The listing builds one solid part. Answer for the finished solid, in the listing's coordinates (mm). A direction names the side the tool comes from. Round coordinates to 2 decimals unless told otherwise and drop trailing zeros. Order: outer loops, then holes, each group sorted by start corner. A loop starts at its lowest first (then second) coordinate and runs counter-clockwise, first axis right, second up. Notation, with made-up numbers: (26.5, 48.25) - (68.5, 48.25) arc R15 ccw to (68.5, 75.25) - close; hole circle Ø9 at (49, 51). An arc over 180 degrees is marked (long way). Use CSV: the item, a comma, the result in double quotes. Start each with the question number.
Item 1: For faces 4 (the flat face through (-1, 53, 2)), 5 (the flat face through (58.1, 4.5, 4.7)), 6 (the flat face through (118, 2, 2)), determine the directions among +Z, -Z, +X, -X, +Y, -Y from which every point of the face is accessible in a straight line to the end or side of a thin tool.
Item 2: Flat-ended cylindrical pins translate along their axes: P1, Ø1, axis at y = 54, z = 1.5, coming from the -X side; P2, Ø2, axis at x = 74, z = 3.5, coming from the +Y side; P3, Ø5, axis at y = 9.5, z = 6, coming from the -X side; P4, Ø8, axis at x = 76, y = 16.5, coming from the -Z side. Find the tip coordinate at first contact, or state that the pin passes through.
Item 3: Determine the mould class of faces 1 (the cylindrical face through (0.738, 53.523, 0.986)), 2 (the flat face through (64, 9, 2)), 3 (the flat face through (53, 8, 24)) for opening direction Z: +Z half, -Z half, draft (parallel to the pull), parting line (faces both ways), or undercut.
Item 4: Find section B-B, the plane x = 93. Give the vertices of the cut face in (y, z), plus the area to 3 significant figures.
Item 5: Find section A-A, the plane y = 31.5. Give the vertices of the cut face in (x, z).
Item 6: Find section C-C, the plane z = 12.75. Give the vertices of the cut face in (x, y), plus the area to 3 significant figures.
Item 7: Straight lines are drawn through the part: line 1 along Z through (x, y) = (68, 6.5); line 2 along Y through (x, z) = (81.5, 22.5); line 3 along X through (y, z) = (22, 22.5). For each, find the intervals that lie inside material, in ascending order. Write a range as [from, to].
```python
from build123d import *

# Parameters (mm, degrees)
SKETCH1_R           = 1.6
SKETCH1_R_2         = 2.1
BOSS_EXTRUDE3_DEPTH = 2
BOSS_EXTRUDE4_DEPTH = 2
SKETCH4_W           = 66
SKETCH4_H           = 16.340111315
SKETCH4_H_2         = 24.741581589
CUT_EXTRUDE3_DEPTH  = 14.5
FILLET1_R           = 4
SKETCH5_W           = 26
SKETCH5_H           = 27
SKETCH5_R           = 6
BOSS_EXTRUDE5_DEPTH = 2
SKETCH6_W           = 5
SKETCH6_H           = 27
CUT_EXTRUDE4_DEPTH  = 14.5
SKETCH7_R           = 1.6
SKETCH7_W           = 110.82382425
SKETCH7_H           = 47.94215156
BOSS_EXTRUDE6_DEPTH = 2
SKETCH8_W           = 110.82382425
SKETCH8_H           = 47.94215156
CUT_EXTRUDE5_DEPTH  = 10
BOSS_EXTRUDE7_DEPTH = 2
BOSS_EXTRUDE8_DEPTH = 21
SKETCH11_W          = 140
SKETCH11_H          = 47.94215156
BOSS_EXTRUDE9_DEPTH = 1
CUT_EXTRUDE7_DEPTH  = 13
CUT_EXTRUDE8_DEPTH  = 13
CUT_EXTRUDE9_DEPTH  = 66
CUT_EXTRUDE11_DEPTH = 66
CUT_EXTRUDE12_DEPTH = 66


with BuildPart() as part:
    # Sketch1 → Boss-Extrude3 (new body)
    with BuildSketch(Plane.XY):
        with BuildLine():
            Line((0, 3.5), (37.911912125, 3.5))
            Line((37.911912125, 3.5), (37.911912125, 13.97107578))
            Line((37.911912125, 13.97107578), (37.911912125, 40.97107578))
            Line((37.911912125, 40.97107578), (37.911912125, 51.44215156))
            Line((37.911912125, 51.44215156), (0, 51.44215156))
            ThreePointArc((0, 51.44215156), (-3.5, 54.94215156), (0, 58.44215156))
            Line((0, 58.44215156), (45.911912125, 58.44215156))
            Line((45.911912125, 58.44215156), (45.911912125, 51.44215156))
            Line((45.911912125, 51.44215156), (45.911912125, 48.97107578))
            Line((45.911912125, 48.97107578), (50.911912125, 48.97107578))
            Line((50.911912125, 48.97107578), (66.911912125, 48.97107578))
            Line((66.911912125, 48.97107578), (71.911912125, 48.97107578))
            Line((71.911912125, 48.97107578), (71.911912125, 51.44215156))
            Line((71.911912125, 51.44215156), (71.911912125, 58.44215156))
            Line((71.911912125, 58.44215156), (117.82382425, 58.44215156))
            ThreePointArc((117.82382425, 58.44215156), (121.32382425, 54.94215156), (117.82382425, 51.44215156))
            Line((117.82382425, 51.44215156), (79.911912125, 51.44215156))
            Line((79.911912125, 51.44215156), (79.911912125, 40.97107578))
            Line((79.911912125, 40.97107578), (79.911912125, 13.97107578))
            Line((79.911912125, 13.97107578), (79.911912125, 3.5))
            Line((79.911912125, 3.5), (117.82382425, 3.5))
            ThreePointArc((117.82382425, 3.5), (121.32382425, 0), (117.82382425, -3.5))
            Line((117.82382425, -3.5), (71.911912125, -3.5))
            Line((71.911912125, -3.5), (71.911912125, 3.5))
            Line((71.911912125, 3.5), (71.911912125, 5.97107578))
            Line((71.911912125, 5.97107578), (66.911912125, 5.97107578))
            Line((66.911912125, 5.97107578), (50.911912125, 5.97107578))
            Line((50.911912125, 5.97107578), (45.911912125, 5.97107578))
            Line((45.911912125, 5.97107578), (45.911912125, 3.5))
            Line((45.911912125, 3.5), (45.911912125, -3.5))
            Line((45.911912125, -3.5), (0, -3.5))
            ThreePointArc((0, -3.5), (-3.5, 0), (0, 3.5))
        make_face()
        with Locations((0, 54.94215156)):
            Circle(SKETCH1_R, mode=Mode.SUBTRACT)
        with Locations((117.82382425, 54.94215156)):
            Circle(SKETCH1_R, mode=Mode.SUBTRACT)
        with Locations((117.82382425, 0)):
            Circle(SKETCH1_R, mode=Mode.SUBTRACT)
        Circle(SKETCH1_R, mode=Mode.SUBTRACT)
        with Locations((66.911912125, 44.97107578)):
            Circle(SKETCH1_R_2, mode=Mode.SUBTRACT)
        with Locations((66.911912125, 9.97107578)):
            Circle(SKETCH1_R_2, mode=Mode.SUBTRACT)
        with Locations((50.911912125, 9.97107578)):
            Circle(SKETCH1_R_2, mode=Mode.SUBTRACT)
        with Locations((50.911912125, 44.97107578)):
            Circle(SKETCH1_R_2, mode=Mode.SUBTRACT)
        Polygon((66.911912125, 40.97107578), (50.911912125, 40.97107578), (45.911912125, 40.97107578), (45.911912125, 27.47107578), (45.911912125, 13.97107578), (50.911912125, 13.97107578), (66.911912125, 13.97107578), (71.911912125, 13.97107578), (71.911912125, 27.47107578), (71.911912125, 40.97107578), align=None, mode=Mode.SUBTRACT)
    extrude(amount=BOSS_EXTRUDE3_DEPTH)

    # Sketch3 → Boss-Extrude4 (add)
    with BuildSketch(Plane.XY.offset(2)):
        Polygon((71.911912125, 13.97107578), (99.911912125, 13.97107578), (99.911912125, 3.5), (91.911912125, 3.5), (91.911912125, 5.97107578), (71.911912125, 5.97107578), align=None)
        Polygon((91.911912125, 51.44215156), (99.911912125, 51.44215156), (99.911912125, 40.97107578), (71.911912125, 40.97107578), (71.911912125, 48.97107578), (91.911912125, 48.97107578), align=None)
        Polygon((45.911912125, 40.97107578), (17.911912125, 40.97107578), (17.911912125, 51.44215156), (25.911912125, 51.44215156), (25.911912125, 48.97107578), (45.911912125, 48.97107578), align=None)
        Polygon((25.911912125, 3.5), (17.911912125, 3.5), (17.911912125, 13.97107578), (45.911912125, 13.97107578), (45.911912125, 5.97107578), (25.911912125, 5.97107578), align=None)
    extrude(amount=-BOSS_EXTRUDE4_DEPTH)

    # Sketch4 → Cut-Extrude3 (cut)
    with BuildSketch(Plane.XY.offset(2)):
        with Locations((58.911912125, 57.141131438)):
            Rectangle(SKETCH4_W, SKETCH4_H)
        with Locations((58.911912125, -6.399715014)):
            Rectangle(SKETCH4_W, SKETCH4_H_2)
    extrude(amount=-CUT_EXTRUDE3_DEPTH, mode=Mode.SUBTRACT)

    # Fillet1
    fillet1_edges = [part.edges().sort_by_distance(p)[0] for p in [
        (99.911912125, 13.97107578, 1),
        (99.911912125, 3.5, 1),
        (91.911912125, 5.97107578, 1),
        (91.911912125, 48.97107578, 1),
        (99.911912125, 51.44215156, 1),
        (99.911912125, 40.97107578, 1),
        (17.911912125, 40.97107578, 1),
        (17.911912125, 51.44215156, 1),
        (25.911912125, 48.97107578, 1),
        (25.911912125, 5.97107578, 1),
        (17.911912125, 3.5, 1),
        (17.911912125, 13.97107578, 1),
        (91.911912125, 58.44215156, 1),
        (25.911912125, 58.44215156, 1),
        (91.911912125, -3.5, 1),
        (25.911912125, -3.5, 1),
    ]]
    fillet(fillet1_edges, radius=FILLET1_R)

    # Sketch5 → Boss-Extrude5 (add)
    with BuildSketch(Plane.XY.offset(2)):
        with Locations((58.911912125, 27.47107578)):
            Rectangle(SKETCH5_W, SKETCH5_H)
        with Locations((58.911912125, 27.47107578)):
            Circle(SKETCH5_R, mode=Mode.SUBTRACT)
    extrude(amount=-BOSS_EXTRUDE5_DEPTH)

    # Sketch6 → Cut-Extrude4 (cut)
    with BuildSketch(Plane.XY.offset(2)):
        with Locations((40.411912125, 27.47107578)):
            Rectangle(SKETCH6_W, SKETCH6_H)
        with Locations((77.411912125, 27.47107578)):
            Rectangle(SKETCH6_W, SKETCH6_H)
    extrude(amount=-CUT_EXTRUDE4_DEPTH, mode=Mode.SUBTRACT)

    # Sketch7 → Boss-Extrude6 (add)
    with BuildSketch(Plane.XY.offset(2)):
        with BuildLine():
            Line((-3.5, 54.94215156), (-3.5, 0))
            ThreePointArc((-3.5, 0), (-2.474873734, -2.474873734), (0, -3.5))
            Line((0, -3.5), (117.82382425, -3.5))
            ThreePointArc((117.82382425, -3.5), (120.298697984, -2.474873734), (121.32382425, 0))
            Line((121.32382425, 0), (121.32382425, 54.94215156))
            ThreePointArc((121.32382425, 54.94215156), (120.298697984, 57.417025294), (117.82382425, 58.44215156))
            Line((117.82382425, 58.44215156), (0, 58.44215156))
            ThreePointArc((0, 58.44215156), (-2.474873734, 57.417025294), (-3.5, 54.94215156))
        make_face()
        Circle(SKETCH7_R, mode=Mode.SUBTRACT)
        with Locations((117.82382425, 0)):
            Circle(SKETCH7_R, mode=Mode.SUBTRACT)
        with Locations((117.82382425, 54.94215156)):
            Circle(SKETCH7_R, mode=Mode.SUBTRACT)
        with Locations((0, 54.94215156)):
            Circle(SKETCH7_R, mode=Mode.SUBTRACT)
        with Locations((58.911912125, 27.47107578)):
            Rectangle(SKETCH7_W, SKETCH7_H, mode=Mode.SUBTRACT)
    extrude(amount=-BOSS_EXTRUDE6_DEPTH)

    # Sketch8 → Cut-Extrude5 (cut)
    with BuildSketch(Plane.XY.offset(2)):
        with Locations((58.911912125, 27.47107578)):
            Rectangle(SKETCH8_W, SKETCH8_H)
    extrude(amount=-CUT_EXTRUDE5_DEPTH, mode=Mode.SUBTRACT)

    # Sketch9 → Boss-Extrude7 (add)
    with BuildSketch(Plane.XY.offset(2)):
        Polygon((58.911912125, 51.44215156), (128.911912125, 51.44215156), (128.911912125, 3.5), (-11.088087875, 3.5), (-11.088087875, 51.44215156), align=None)
    extrude(amount=-BOSS_EXTRUDE7_DEPTH)

    # Sketch10 → Boss-Extrude8 (add)
    with BuildSketch(Plane.XY.offset(2)):
        Polygon((-11.088087875, 51.44215156), (128.911912125, 51.44215156), (128.911912125, 3.5), (-11.088087875, 3.5), (-11.088087875, 4.5), (127.911912125, 4.5), (127.911912125, 27.47107578), (127.911912125, 50.44215156), (-11.088087875, 50.44215156), align=None)
    extrude(amount=BOSS_EXTRUDE8_DEPTH)

    # Sketch11 → Boss-Extrude9 (add)
    with BuildSketch(Plane.XY.offset(23)):
        with Locations((58.911912125, 27.47107578)):
            Rectangle(SKETCH11_W, SKETCH11_H)
    extrude(amount=BOSS_EXTRUDE9_DEPTH)

    # Sketch12 → Cut-Extrude7 (cut)
    with BuildSketch(Plane.XY.offset(2)):
        with BuildLine():
            Line((3.5, 0), (3.5, 3.5))
            Line((3.5, 3.5), (114.32382425, 3.5))
            Line((114.32382425, 3.5), (114.32382425, 0))
            ThreePointArc((114.32382425, 0), (115.348950516, -2.474873734), (117.82382425, -3.5))
            Line((117.82382425, -3.5), (0, -3.5))
            ThreePointArc((0, -3.5), (2.474873734, -2.474873734), (3.5, 0))
        make_face()
        with BuildLine():
            Line((3.5, 54.94215156), (3.5, 51.44215156))
            Line((3.5, 51.44215156), (114.32382425, 51.44215156))
            Line((114.32382425, 51.44215156), (114.32382425, 54.94215156))
            ThreePointArc((114.32382425, 54.94215156), (115.348950516, 57.417025294), (117.82382425, 58.44215156))
            Line((117.82382425, 58.44215156), (0, 58.44215156))
            ThreePointArc((0, 58.44215156), (2.474873734, 57.417025294), (3.5, 54.94215156))
        make_face()
    extrude(amount=-CUT_EXTRUDE7_DEPTH, mode=Mode.SUBTRACT)

    # Sketch13 → Cut-Extrude8 (cut)
    with BuildSketch(Plane(origin=(128.911912125, 0, 0), x_dir=(0, 0, -1), z_dir=(1, 0, 0))):
        Polygon((-20, 27.47107578), (-20, 47.44215156), (-5, 47.44215156), (-5, 7.5), (-20, 7.5), align=None)
    extrude(amount=-CUT_EXTRUDE8_DEPTH, mode=Mode.SUBTRACT)

    # Sketch14 → Cut-Extrude9 (cut)
    with BuildSketch(Plane(origin=(0, 0, 0), x_dir=(-1, 0, 0), z_dir=(0, 0, -1))):
        Polygon((-58.911912125, 9.5), (-122.911912125, 9.5), (-122.911912125, 45.44215156), (5.088087875, 45.44215156), (5.088087875, 9.5), align=None)
    extrude(amount=-CUT_EXTRUDE9_DEPTH, mode=Mode.SUBTRACT)

    # Sketch15 → Cut-Extrude11 (cut)
    with BuildSketch(Plane(origin=(0, 51.44215156, 0), x_dir=(1, 0, 0), z_dir=(0, 1, 0))):
        Polygon((-1.088087875, -5), (-1.088087875, -12), (-1.088087875, -20), (124.911912125, -20), (124.911912125, -5), (58.911912125, -5), align=None)
    extrude(amount=-CUT_EXTRUDE11_DEPTH, mode=Mode.SUBTRACT)

    # Sketch16 → Cut-Extrude12 (cut)
    with BuildSketch(Plane(origin=(0, 51.44215156, 0), x_dir=(1, 0, 0), z_dir=(0, 1, 0))):
        Polygon((-6.088087875, -12), (-6.088087875, -5), (-11.088087875, -5), (-11.088087875, -20), (-6.088087875, -20), align=None)
    extrude(amount=-CUT_EXTRUDE12_DEPTH, mode=Mode.SUBTRACT)


solid = part.part
```
Worked out:
1,face 4,"+Z, +X, -X, +Y"
1,face 5,"-X"
1,face 6,"+Z, +X, -X, -Y"
2,P1,"stops at x = -3.5"
2,P2,"stops at y = 51.44"
2,P3,"stops at x = 127.91"
2,P4,"passes through"
3,face 1,"draft"
3,face 2,"undercut"
3,face 3,"+Z half"
4,outline,"(3.5, 0) - (9.5, 0) - (9.5, 2) - (4.5, 2) - (4.5, 5) - (3.5, 5) - close; (3.5, 20) - (4.5, 20) - (4.5, 23) - (9.5, 23) - (9.5, 24) - (3.5, 24) - close; (45.44, 0) - (51.44, 0) - (51.44, 5) - (50.44, 5) - (50.44, 2) - (45.44, 2) - close; (45.44, 23) - (50.44, 23) - (50.44, 20) - (51.44, 20) - (51.44, 24) - (45.44, 24) - close"
4,area,"48.0 mm²"
5,outline,"(-11.09, 0) - (-5.09, 0) - (-5.09, 2) - (-11.09, 2) - close; (-11.09, 23) - (-5.09, 23) - (-5.09, 24) - (-11.09, 24) - close; (122.91, 0) - (128.91, 0) - (128.91, 5) - (127.91, 5) - (127.91, 2) - (122.91, 2) - close; (122.91, 23) - (127.91, 23) - (127.91, 20) - (128.91, 20) - (128.91, 24) - (122.91, 24) - close"
6,outline,"(-6.09, 3.5) - (-1.09, 3.5) - (-1.09, 4.5) - (-6.09, 4.5) - close; (-6.09, 50.44) - (-1.09, 50.44) - (-1.09, 51.44) - (-6.09, 51.44) - close; (124.91, 3.5) - (128.91, 3.5) - (128.91, 7.5) - (127.91, 7.5) - (127.91, 4.5) - (124.91, 4.5) - close; (124.91, 50.44) - (127.91, 50.44) - (127.91, 47.44) - (128.91, 47.44) - (128.91, 51.44) - (124.91, 51.44) - close"
6,area,"24.0 mm²"
7,line 1,"z = [0, 2], [23, 24]"
7,line 2,"y = [3.5, 4.5], [50.44, 51.44]"
7,line 3,"x = [127.91, 128.91]"
